from build123d import *

# Parameters (mm, degrees)
CROQUIS1_R              = 5
CROQUIS1_R_2            = 1
SALIENTE_EXTRUIR1_DEPTH = 5
REDONDEO1_R             = 2


with BuildPart() as part:
    # Croquis1 → Saliente-Extruir1 (new body)
    with BuildSketch(Plane(origin=(0, 0, 0), x_dir=(1, 0, 0), z_dir=(0, 1, 0))):
        with BuildLine():
            Line((125, -9), (125, 9))
            Line((125, 9), (0, 11.4))
            ThreePointArc((0, 11.4), (-11.4, 0), (0, -11.4))
            Line((0, -11.4), (125, -9))
        make_face()
        with Locations(Location((115, 0, 0), (0, 0, 270))):
            Circle(CROQUIS1_R, mode=Mode.SUBTRACT)
        with Locations(Location((-8, -0.055168642, 0), (0, 0, 270))):
            Circle(CROQUIS1_R_2, mode=Mode.SUBTRACT)
        with Locations(Location((0, -8, 0), (0, 0, 270))):
            Circle(CROQUIS1_R_2, mode=Mode.SUBTRACT)
        with Locations(Location((0, 8, 0), (0, 0, 270))):
            Circle(CROQUIS1_R_2, mode=Mode.SUBTRACT)
        with Locations(Location((8, 0, 0), (0, 0, 270))):
            Circle(CROQUIS1_R_2, mode=Mode.SUBTRACT)
    extrude(amount=SALIENTE_EXTRUIR1_DEPTH)

    # Redondeo1
    redondeo1_edges = [part.edges().sort_by_distance(p)[0] for p in [
        (125, 2.5, -9),
        (125, 2.5, 9),
    ]]
    fillet(redondeo1_edges, radius=REDONDEO1_R)


solid = part.part
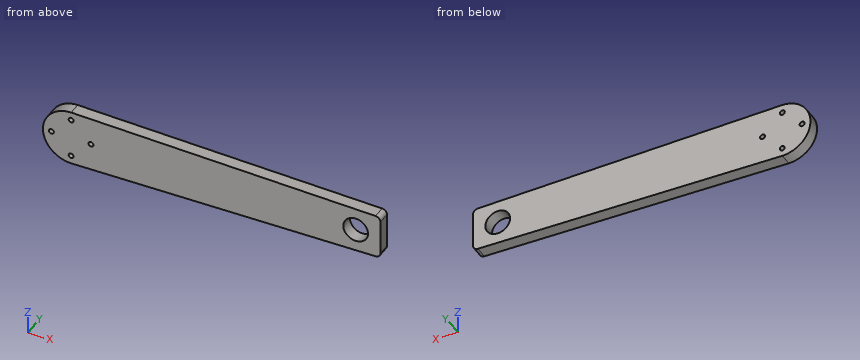
Here's how the part is built. I have some questions about the finished solid (model axes, mm). Coordinates: 2 decimals unless noted, no trailing zeros. Loops run counter-clockwise (first coordinate to the right, second up) from the corner with the lowest first, then second, coordinate; pieces in that order, holes last.
1. For P1, Ø1, axis at x = 50.5, y = 2.5, coming from the +Z side; P2, Ø1, axis at x = 35.5, y = 4.5, coming from the -Z side; P3, Ø3, axis at x = 8.5, y = 1, coming from the -Z side, each with a flat end and sliding along its axis, tell me the tip position at first contact or that it passes through.
2. Imagine slicing it at B-B, the plane x = 115. Please give me the cut outline in (y, z), and give its area (3 significant figures).
3. Imagine slicing it at A-A, the plane y = 4. Please give me the cut outline in (x, z).
4. I need wall thicknesses on L1, parallel to X at y = 3.3, z = 0; L2, parallel to X at y = 1.25, z = -8; L3, parallel to X at y = 2.6, z = -3. Which ranges of each line are inside material? Lowest first, please.
5. Imagine slicing it at C-C, the plane z = -3.75. Please give me the cut outline in (x, y).
6. Imagine slicing it at D-D, the plane x = 51.5. Please give me the cut outline in (y, z), and give its area (3 significant figures).
Taken from the geometry:
1. P1: stops at z = 10.44
1. P2: stops at z = -10.73
1. P3: stops at z = -11.27
2. outline: (0, -9.19) - (5, -9.19) - (5, -5) - (0, -5) - close; (0, 5) - (5, 5) - (5, 9.19) - (0, 9.19) - close
2. area: 41.9 mm2
3. outline: (0, -11.4) - (123.04, -9.04) arc R2 ccw to (125, -7.04) - (125, 7.04) arc R2 ccw to (123.04, 9.04) - (0, 11.4) arc R11.4 ccw to start; hole circle Ø2 at (-8, 0.06); hole circle Ø2 at (0, -8); hole circle Ø2 at (0, 8); hole circle Ø2 at (8, 0); hole circle Ø10 at (115, 0)
4. L1: x = -11.4 to -9, -7 to 7, 9 to 110, 120 to 125
4. L2: x = -8.12 to -1, 1 to 124.75
4. L3: x = -11 to 111, 119 to 125
5. outline: (-10.77, 0) - (111.69, 0) - (111.69, 5) - (-10.77, 5) - close; (118.31, 0) - (125, 0) - (125, 5) - (118.31, 5) - close
6. outline: (0, -10.41) - (5, -10.41) - (5, 10.41) - (0, 10.41) - close
6. area: 104 mm2
